from build123d import *

# Parameters (mm, degrees)
F1_DEPTH       = 101.6
F5_DEPTH       = 50
F7_D           = 9
F7_DEPTH       = 12
F7_CBORE_D     = 14.25
F7_CBORE_DEPTH = 8
F7_TIP         = 2.7038727856


with BuildPart() as f1:
    # F0 (on Top) → F1 (new body)
    with BuildSketch(Plane.XY):
        Polygon((-109.12142694, 45.1170913875), (-104.8183739185, -41.8617390096), (27.9122088104, -41.8617390096), (27.9122088104, 45.1170913875), align=None)
    extrude(amount=F1_DEPTH)

    # F2 (on face) → F3 (revolve)
    with BuildSketch(Plane.XZ.offset(41.8617390096)):
        Polygon((-104.8183739185, 0), (-104.8183739185, 50.8), (-134.8183739185, 50.8), (-107.7620375156, 0), align=None)
    revolve(axis=Axis((27.9122088104, -41.8617390096, 50.8), (0, 0, -1)))

    # F4 (on face) → F5 (intersect)
    with BuildSketch(Plane.XY.offset(101.6)):
        Polygon((27.9122088104, 45.1170913875), (-109.12142694, 45.1170913875), (-104.8183739185, -41.8617390096), (27.9122088104, -41.8617390096), align=None)
        Polygon((-51.6147029857, -9.5938752115), (-40.3364262624, 25.1170913875), (-3.8391561167, 25.1170913875), (7.4391206066, -9.5938752115), (-22.0877911896, -31.046432352), align=None, mode=Mode.SUBTRACT)
    extrude(amount=-F5_DEPTH, mode=Mode.INTERSECT)

    # F7
    with Locations(Plane.XY.offset(101.6)):
        with Locations((-82.40018785, -16.1850638688), (-84.7880318761, 7.7034095302), (-77.399738133, 22.8778515011)):
            CounterBoreHole(F7_D / 2, F7_CBORE_D / 2, F7_CBORE_DEPTH, depth=F7_DEPTH)
            with Locations((0, 0, -(F7_DEPTH + F7_TIP / 2))):  # 118° drill point
                Cone(0, F7_D / 2, F7_TIP, mode=Mode.SUBTRACT)


solid = f1.part
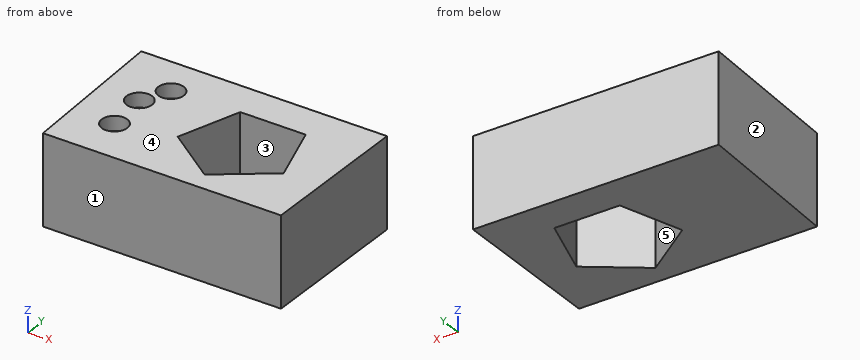
The listing builds one solid part. Answer for the finished solid, in the listing's coordinates (mm). Face numbers are marked on the shaded views. A direction names the side the tool comes from. Round coordinates to 2 decimals unless told otherwise and drop trailing zeros. Loops run counter-clockwise (first coordinate to the right, second up) from the corner with the lowest first, then second, coordinate; pieces in that order, holes last. Notation, with made-up numbers: M 17.5,88 L 29.5,88 A20 ccw 29.5,97 Z; hole C 85,27 d9. An arc over 180 degrees is marked long. Return JSON: item names as keys, results as strings.
Q1. Which of the six approach directions +Z, -Z, +X, -X, +Y, -Y give full straight-line access (tool end or side, diameter ignored) to the marked faces 4 and 5?
Results list:
{"face 4": "+Z, +X, -X, +Y, -Y", "face 5": "+Z, -Z"}
Q2. Each of these flat-tipped pins is pushed along its axis until it touches: pin 1 Ø4.5 at (x, y) = (-87, 11) entering from +Z; pin 2 Ø8.5 at (x, y) = (-84.79, 7.7) entering from +Z; pin 3 Ø2 at (y, z) = (-23, 64) entering from -X. Where does it stop, or does it pass through?
Results list:
{"pin 1": "stops at z = 93.6", "pin 2": "stops at z = 89.45", "pin 3": "stops at x = -105.8"}
Q3. Find section B-B, the plane x = -32.5. Determine the outline of the cut face in (y, z), plus the area to 3 significant figures.
Results list:
{"outline": "M -41.86,51.6 L -23.48,51.6 L -23.48,101.6 L -41.86,101.6 Z; M 25.12,51.6 L 45.12,51.6 L 45.12,101.6 L 25.12,101.6 Z", "area": "1,920 mm2"}
Q4. Find section D-D, the plane z = 96. Determine the outline of the cut face in (x, y) (3 decimals), plus the area to 3 significant figures.
Results list:
{"outline": "M -109.121,45.117 L -104.818,-41.862 L 27.912,-41.862 L 27.912,45.117 Z; hole C -84.788,7.703 d14.25; hole C -82.4,-16.185 d14.25; hole C -77.4,22.878 d14.25; hole M -51.615,-9.594 L -22.088,-31.046 L 7.439,-9.594 L -3.839,25.117 L -40.336,25.117 Z", "area": "8,960 mm2"}
Q5. Find the intervals of material crossed by line 1 along X through (y, z) = (20, 97); line 2 along X through (y, z) = (17, 96); line 3 along X through (y, z) = (-17.5, 87), in increasing order. Write a range as from..to.
Results list:
{"line 1": "x = -107.88..-83.92, -70.88..-42, -2.18..27.91", "line 2": "x = -107.73..-81.43, -73.37..-42.97, -1.2..27.91", "line 3": "x = -106.02..-40.73, -3.44..27.91"}
Q6. Find section A-A, the plane z = 85. Determine the outline of the cut face in (x, y), plus the area to 3 significant figures.
Results list:
{"outline": "M -109.12,45.12 L -104.82,-41.86 L 27.91,-41.86 L 27.91,45.12 Z; hole M -51.61,-9.59 L -22.09,-31.05 L 7.44,-9.59 L -3.84,25.12 L -40.34,25.12 Z", "area": "9,440 mm2"}
Q7. Find section C-C, the plane y = -26. Determine the outline of the cut face in (x, z), plus the area to 3 significant figures.
Results list:
{"outline": "M -105.6,51.6 L -29.03,51.6 L -29.03,101.6 L -105.6,101.6 Z; M -15.14,51.6 L 27.91,51.6 L 27.91,101.6 L -15.14,101.6 Z", "area": "5,980 mm2"}
Q8. The mould has two halves that part along X. Classify the marked faces 1, 2 and 3: released by +X, released by -X, zero draft, split by the parting line, or undercut.
Results list:
{"face 1": "zero draft", "face 2": "released by -X", "face 3": "undercut"}
